Read the model definition and answer for the solid it produces. Units are mm, in the model's axes. A direction names the side the tool comes from. Round coordinates to 2 decimals unless told otherwise and drop trailing zeros. Order: outer loops, then holes, each group sorted by start corner. A loop starts at its lowest first (then second) coordinate and runs counter-clockwise, first axis right, second up.
from build123d import *

# Parameters (mm, degrees)
F0_W     = 96.628905
F0_H     = 101.417847
F1_DEPTH = 127
F3_DEPTH = 127


with BuildPart() as f1:
    # F0 (on Front) → F1 (new body)
    with BuildSketch(Plane.XZ):
        with Locations((6.532389, 10.024552)):
            Rectangle(F0_W, F0_H)
    extrude(amount=F1_DEPTH)

    # F2 (on Front) → F3 (join)
    with BuildSketch(Plane.XZ):
        Polygon((-86.055711, -80.979206), (143.171892, -80.979206), (28.55809, 117.537722), align=None)
    extrude(amount=F3_DEPTH)


solid = f1.part
Q1. A cutting plane is placed at A-A, the plane y = -105. Give the vertices of the cut face in (x, z) (3 decimals), plus the area to 3 significant figures.
Outcome:
outline: (-86.056, -80.979) - (143.172, -80.979) - (28.558, 117.538) - (-4.238, 60.733) - (-41.782, 60.733) - (-41.782, -4.295) - close
area: 24,000 mm2
Q2. For faces 1 (the face through (27, -63, -80.979)), 2 (the face through (-41.782, -63, 28)), determine the directions among +Z, -Z, +X, -X, +Y, -Y from which every point of the face is accessible in a straight line to the end or side of a thin tool.
Outcome:
face 1: -Z, +X, -X, +Y, -Y
face 2: +Z, -X, +Y, -Y
Q3. A cutting plane is placed at C-C, the plane x = 59. Give the vertices of the cut face in (y, z), plus the area to 3 significant figures.
Outcome:
outline: (-127, -80.98) - (0, -80.98) - (0, 64.81) - (-127, 64.81) - close
area: 18,500 mm2
Q4. A cutting plane is placed at B-B, the plane z = 25. Give the vertices of the cut face in (x, y), plus the area to 3 significant figures.
Outcome:
outline: (-41.78, -127) - (81.98, -127) - (81.98, 0) - (-41.78, 0) - close
area: 15,700 mm2
Q5. Flat-ended cylindrical pins translate along their axes: pin 1 (3 mm diameter, centred on y = -51, z = 46.5, fed in from -X); pin 2 (19 mm diameter, centred on x = -19, y = -83, fed in from +Z); pin 3 (4 mm diameter, centred on x = 59.5, y = -69.5, fed in from +Z). Find the tip coordinate at first contact, or state that the pin passes through.
Outcome:
pin 1: stops at x = -41.78
pin 2: stops at z = 60.73
pin 3: stops at z = 67.41
Q6. Straight lines are drawn through the part: probe 1 along Z at (x, y) = (-25, -109); probe 2 along Z at (x, y) = (-45, -96.5); probe 3 along X at (y, z) = (-65.5, -6). For each, find the intervals that lie inside material, in ascending order.
Outcome:
probe 1: z = -80.98 to 60.73
probe 2: z = -80.98 to -9.87
probe 3: x = -42.77 to 99.88
